Here's the drawing with two shaded views (mm, measured from the low corner). I have some questions. Coordinates: 2 decimals unless noted, no trailing zeros. Write each loop counter-clockwise with the first axis right and the second up, starting at its lowest first coordinate (ties: lowest second). Pieces come first, ordered by that corner, then holes. Notation, with made-up numbers: (14, 79) - (66, 79) arc R14 cw to (66, 89) - close; hole circle Ø5 at (-39, 63.25). An arc over 180 degrees is marked (long way). Answer in a Markdown table with one row per item. Add a question column.
Item 1: Imagine slicing it at C-C (x = 7). Please give me the cut outline in (y, z), plus the area to 3 significant figures.
Item 2: Imagine slicing it at A-A (y = 6). Please give me the cut outline in (x, z).
Item 3: We'd pull the mould along Y, two halves only. Please class the marked faces 1, 2 and 3: +Y half, -Y half, draft (parallel to the pull), parting line (faces both ways), or undercut.
Item 4: I'm going to push flat-ended pins straight in: pin 1 (1 mm diameter, centred on x = 52.5, y = 6.5, fed in from +Z); pin 2 (5 mm diameter, centred on x = 7, y = 6, fed in from +Z). Where does each tip first touch, or does it pass through?
Item 5: Imagine slicing it at B-B (z = 2.1). Please give me the cut outline in (x, y).
Item 6: If I drill on probe 1 along X at (y, z) = (6, 0.45); probe 2 along Y at (x, z) = (53, 0.45); probe 3 along X at (y, z) = (5, 2.7), over which ranges is the centre line in solid material (lowest first)? Write a range as from..to.
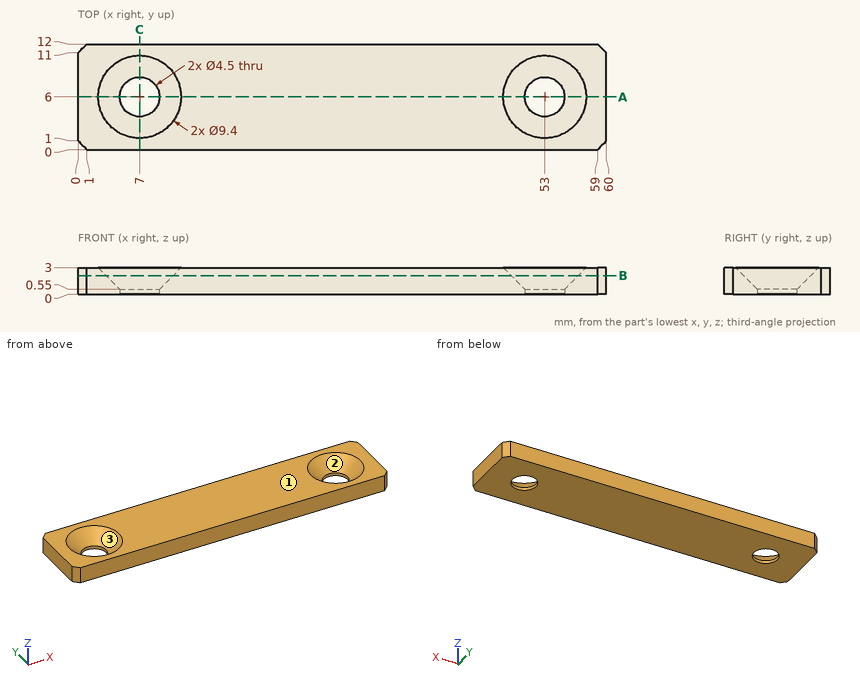
Here are the results:
| question | item | result |
|---|---|---|
| 1 | outline | (0, 0) - (3.75, 0) - (3.75, 0.55) - (1.3, 3) - (0, 3) - close; (8.25, 0) - (12, 0) - (12, 3) - (10.7, 3) - (8.25, 0.55) - close |
| 1 | area | 16.5 mm2 |
| 2 | outline | (0, 0) - (4.75, 0) - (4.75, 0.55) - (2.3, 3) - (0, 3) - close; (9.25, 0) - (50.75, 0) - (50.75, 0.55) - (48.3, 3) - (11.7, 3) - (9.25, 0.55) - close; (55.25, 0) - (60, 0) - (60, 3) - (57.7, 3) - (55.25, 0.55) - close |
| 3 | face 1 | draft |
| 3 | face 2 | undercut |
| 3 | face 3 | undercut |
| 4 | pin 1 | passes through |
| 4 | pin 2 | stops at z = 0.8 |
| 5 | outline | (0, 1) - (1, 0) - (59, 0) - (60, 1) - (60, 11) - (59, 12) - (1, 12) - (0, 11) - close; hole circle Ø7.6 at (7, 6); hole circle Ø7.6 at (53, 6) |
| 6 | probe 1 | x = 0..4.75, 9.25..50.75, 55.25..60 |
| 6 | probe 2 | y = 0..3.75, 8.25..12 |
| 6 | probe 3 | x = 0..2.72, 11.28..48.72, 57.28..60 |
